Autodesk Inventor part; units mm, degrees
ref_plane "YZ Plane" through (0, 0, 0) normal (1, 0, 0) x (0, 1, 0)
ref_plane "XZ Plane" through (0, 0, 0) normal (0, 1, 0) x (-1, 0, 0)
ref_plane "XY Plane" through (0, 0, 0) normal (0, 0, 1) x (1, 0, 0)
sketch "草图1" plane through (0, 0, 0) normal (0, 1, 0) x (-1, 0, 0)
  line L0 (0, 0) -> (15, 0)
  line L1 (15, 0) -> (15, -161)
  line L2 (15, -161) -> (0, -161)
  line L3 (0, -161) -> (0, 0)
  dimension "d0" = 161
  dimension "d1" = 15
extrude "拉伸1" add sketch "草图1" along normal blind 5
sketch "草图2" plane through (-15, 0, -161) normal (-1, 0, 0) x (0, 0, 1)
  line L0 (161, 0) -> (161, 5)
  line L1 (161, 2.5) -> (159, 2.5)
  circle A0 centre (159, 2.5) radius 1.5
  line L2 (159, 2.5) -> (155, 2.5)
  circle A1 centre (155, 2.5) radius 1.5
  dimension "d4" = 2
  dimension "d5" = 3
  dimension "d6" = 4
  dimension "d7" = 3
extrude "拉伸2" cut sketch "草图2" against normal through all
equation "\"折弯半径\" = 厚度"
equation "\"折弯释压宽度\" = 厚度"
equation "\"折弯释压深度\" = 0.5 * 厚度"
equation "\"拐角释压尺寸\" = 4 * 厚度"
equation "\"最小余量\" = 2 * 厚度"
equation "\"过渡半径\" = 折弯半径"
equation "\"Jacobi半径尺寸\" = 折弯半径"
equation "\"间隙大小\" = 厚度"
properties part number "123"
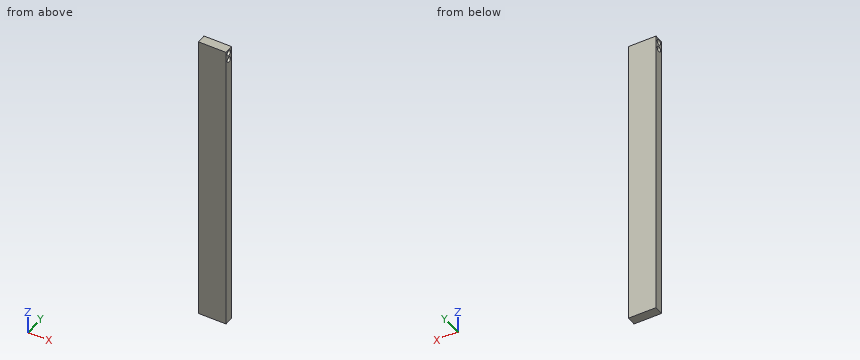
Check sheet for the modelled part. Datum: model origin and axes. Units: mm. Round coordinates to 2 decimals unless told otherwise and drop trailing zeros. Loops run counter-clockwise (first coordinate to the right, second up) from the corner with the lowest first, then second, coordinate; pieces in that order, holes last. Notation, with made-up numbers: (-10, -18.5) - (31, -18.5) arc R18 ccw to (31, 3.5) - close; hole circle Ø3 at (-39, 31). An arc over 180 degrees is marked (long way). Answer as a JSON object with one key per item and string values. Group by question number.
Q1. Sectioned sample at C-C, the plane x = -3.25. Enter the section's corners in (y, z).
Q2. Gauge pin test, flat end, axial feed: P1, Ø3, axis at x = -4, z = -58, coming from the -Y side. Record the tip position at first contact, or that the pin passes through.
Q3. Sectioned sample at B-B, the plane y = 2.5. Enter the section's corners in (x, z), plus the area to 4 significant figures.
Q4. Sectioned sample at A-A, the plane z = -2. Enter the section's corners in (x, y).
Q5. Scan lines: line 1 along Z through (x, y) = (-5.25, 2.25); line 2 along Y through (x, z) = (-12, -2); line 3 along Z through (x, y) = (-10, 3.85). Record each from-to range of solid material in increasing order. Write a range as [from, to].
Solution:
{
 "1": {"outline": "(0, -161) - (5, -161) - (5, 0) - (0, 0) - close; hole circle Ø3 at (2.5, -6); hole circle Ø3 at (2.5, -2)"},
 "2": {"P1": "stops at y = 0"},
 "3": {"outline": "(-15, -161) - (0, -161) - (0, -7.5) - (-15, -7.5) - close; (-15, -4.5) - (0, -4.5) - (0, -3.5) - (-15, -3.5) - close; (-15, -0.5) - (0, -0.5) - (0, 0) - (-15, 0) - close", "area": "2,325 mm²"},
 "4": {"outline": "(-15, 0) - (0, 0) - (0, 1) - (-15, 1) - close; (-15, 4) - (0, 4) - (0, 5) - (-15, 5) - close"},
 "5": {"line 1": "z = [-161, -7.48], [-4.52, -3.48], [-0.52, 0]", "line 2": "y = [0, 1], [4, 5]", "line 3": "z = [-161, -6.65], [-5.35, -2.65], [-1.35, 0]"}
}
